from build123d import *

# Parameters (mm, degrees)
F1_W      = 139.7
F1_H      = 241.3
F2_DEPTH  = 12.7
F4_D      = 14.2875
F5_W      = 139.7
F5_H      = 203.2
F6_DEPTH  = 12.7
F8_DEPTH  = 25.4
F10_DEPTH = 6.35


# Not quite as in the source:
# - a length typed as a fraction of an inch, garbled in the dataset ("3 / 203.2 mm" for 3/8 in), is restored


with BuildPart() as f2:
    # F1 (on Top) → F2 (new body)
    with BuildSketch(Plane.XY):
        Rectangle(F1_W, F1_H)
    extrude(amount=F2_DEPTH)

    # F4 (through all)
    with Locations(Plane.XY.offset(12.7)):
        with Locations((-50.8, 63.5), (50.8, 63.5), (50.8, -63.5), (-50.8, -63.5)):
            Hole(F4_D / 2)



with BuildPart() as f6:
    # F5 (on offset) → F6 (new body)
    with BuildSketch(Plane.XY.offset(250.825)):
        with Locations((19.05, 0)):
            Rectangle(F5_W, F5_H)
    extrude(amount=-F6_DEPTH)

    # F7 (on face) → F8 (cut)
    with BuildSketch(Plane.XY.offset(250.825)):
        with BuildLine():
            ThreePointArc((-26.162, -57.912), (-31.75, -63.5), (-26.162, -69.088))
            Line((-26.162, -69.088), (-11.938, -69.088))
            ThreePointArc((-11.938, -69.088), (-6.35, -63.5), (-11.938, -57.912))
            Line((-11.938, -57.912), (-26.162, -57.912))
        make_face()
        with BuildLine():
            Line((50.038, -69.088), (64.262, -69.088))
            ThreePointArc((64.262, -69.088), (69.85, -63.5), (64.262, -57.912))
            Line((64.262, -57.912), (50.038, -57.912))
            ThreePointArc((50.038, -57.912), (44.45, -63.5), (50.038, -69.088))
        make_face()
        with BuildLine():
            ThreePointArc((64.262, 57.912), (69.85, 63.5), (64.262, 69.088))
            Line((64.262, 69.088), (50.038, 69.088))
            ThreePointArc((50.038, 69.088), (44.45, 63.5), (50.038, 57.912))
            Line((50.038, 57.912), (64.262, 57.912))
        make_face()
        with BuildLine():
            Line((-11.938, 69.088), (-26.162, 69.088))
            ThreePointArc((-26.162, 69.088), (-31.75, 63.5), (-26.162, 57.912))
            Line((-26.162, 57.912), (-11.938, 57.912))
            ThreePointArc((-11.938, 57.912), (-6.35, 63.5), (-11.938, 69.088))
        make_face()
    extrude(amount=-F8_DEPTH, mode=Mode.SUBTRACT)


with BuildPart() as f2_1:
    add(f2.part)

    add(f6.part)  # F10 merges F6
    # F9 (on face) → F10 (join, symmetric)
    with BuildSketch(Plane.XZ.offset(101.6)):
        Polygon((88.9, 238.125), (-50.8, 238.125), (-69.85, 12.7), (69.85, 12.7), align=None)
    extrude(amount=F10_DEPTH, both=True)

    # F11: F2 across plane


with BuildPart() as f2_2:
    add(f2_1.part)
    add(f2_1.part.mirror(Plane.XZ))


solid = f2_2.part
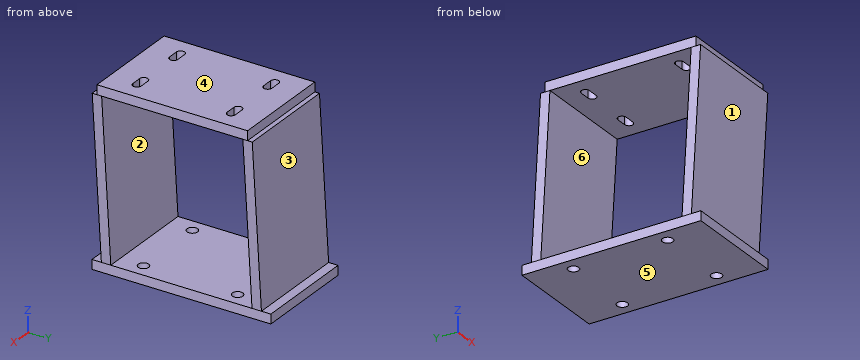
Can you work these out from the model? Positions are in its coordinate system, mm. Face numbers are marked on the shaded views. A direction names the side the tool comes from. Coordinates: 2 decimals unless noted, no trailing zeros. Write each loop counter-clockwise with the first axis right and the second up, starting at its lowest first coordinate (ties: lowest second). Pieces come first, ordered by that corner, then holes. Notation, with made-up numbers: M 89,-0.75 L 103,-0.75 A10 cw 103,4.25 Z; hole C -28,79.5 d11. An arc over 180 degrees is marked long. Use one line per item in the form item = value.
Q1. For the marked faces 1, 2 and 3, which set-ups out of +Z, -Z, +X, -X, +Y, -Y let a thin tool reach every point of the face, with its end or its side?
Model answer:
face_1 = +Z, +X, -X, -Y
face_2 = +X, -X
face_3 = +Z, +X, -X, +Y
Q2. If we section it at B-B (x = 10): Write out the boundary of the cut face in (y, z) (3 decimals), then the cut area to 3 significant figures.
Model answer:
outline = M -120.65,0 L 120.65,0 L 120.65,12.7 L 107.95,12.7 L 107.95,238.125 L 101.6,238.125 L 101.6,250.825 L -101.6,250.825 L -101.6,238.125 L -107.95,238.125 L -107.95,12.7 L -120.65,12.7 Z; hole M -95.25,12.7 L 95.25,12.7 L 95.25,238.125 L -95.25,238.125 Z
area = 11,400 mm^2
Q3. For P1, Ø3, axis at x = 3.5, y = -105, coming from the +Z side (3 decimals); P2, Ø4, axis at x = -19.5, z = 244.5, coming from the -Y side; P3, Ø10, axis at y = -41, z = 246.5, coming from the -X side, each with a flat end and sliding along its axis, tell me the tip position at first contact or that it passes through.
Model answer:
P1 = 238.125
P2 = -101.6
P3 = -50.8
Q4. If we section it at D-D (z = 44): Write out the boundary of the cut face in (x, y), then the cut area to 3 significant figures.
Model answer:
outline = M -67.2,-107.95 L 72.5,-107.95 L 72.5,-95.25 L -67.2,-95.25 Z; M -67.2,95.25 L 72.5,95.25 L 72.5,107.95 L -67.2,107.95 Z
area = 3,550 mm^2
Q5. If we section it at C-C (y = -31): Write out the boundary of the cut face in (x, z) (3 decimals), then the cut area to 3 significant figures.
Model answer:
outline = M -69.85,0 L 69.85,0 L 69.85,12.7 L -69.85,12.7 Z; M -50.8,238.125 L 88.9,238.125 L 88.9,250.825 L -50.8,250.825 Z
area = 3,550 mm^2
Q6. We'd pull the mould along Z, two halves only. Please class the marked faces 4, 5 and 6: +Z half, -Z half, draft (parallel to the pull), parting line (faces both ways), or undercut.
Model answer:
face_4 = +Z half
face_5 = -Z half
face_6 = undercut
Q7. If we section it at A-A (y = 63.5): Write out the boundary of the cut face in (x, z) (3 decimals), then the cut area to 3 significant figures.
Model answer:
outline = M -69.85,0 L -57.944,0 L -57.944,12.7 L -69.85,12.7 Z; M -50.8,238.125 L -31.75,238.125 L -31.75,250.825 L -50.8,250.825 Z; M -43.656,0 L 43.656,0 L 43.656,12.7 L -43.656,12.7 Z; M -6.35,238.125 L 44.45,238.125 L 44.45,250.825 L -6.35,250.825 Z; M 57.944,0 L 69.85,0 L 69.85,12.7 L 57.944,12.7 Z; M 69.85,238.125 L 88.9,238.125 L 88.9,250.825 L 69.85,250.825 Z
area = 2,540 mm^2
Q8. I need wall thicknesses on line 1 along Y through (x, z) = (50.8, 5.25); line 2 along Z through (x, y) = (-30, -30.5) (3 decimals); line 3 along Y through (x, z) = (70, 28). Which ranges of each line are inside material? Lowest first, please. Write a range as from..to.
Model answer:
line_1 = -120.65..-70.64, -56.36..56.36, 70.64..120.65
line_2 = 0..12.7, 238.125..250.825
line_3 = -107.95..-95.25, 95.25..107.95
